from build123d import *

# Parameters (mm, degrees)
SKETCH1_W           = 25.4
SKETCH1_H           = 31.75
BOSS_EXTRUDE1_DEPTH = 25.4
SKETCH2_W           = 3.048
SKETCH2_H           = 19.304
CUT_EXTRUDE1_DEPTH  = 33.534068682
FILLET1_R           = 2.54
CHAMFER1_SIZE       = 1.27


with BuildPart() as part:
    # Sketch1 → Boss-Extrude1 (new body)
    with BuildSketch(Plane(origin=(0, 0, 0), x_dir=(1, 0, 0), z_dir=(0, 1, 0))):
        Rectangle(SKETCH1_W, SKETCH1_H)
    extrude(amount=BOSS_EXTRUDE1_DEPTH)

    # Sketch2 → Cut-Extrude1 (cut, through all)
    with BuildSketch(Plane(origin=(0, 25.4, 0), x_dir=(1, 0, 0), z_dir=(0, 1, 0))):
        with Locations((-4.826, 0)):
            Rectangle(SKETCH2_W, SKETCH2_H)
    extrude(amount=-CUT_EXTRUDE1_DEPTH, mode=Mode.SUBTRACT)

    # Fillet1
    fillet1_edges = [part.edges().sort_by_distance(p)[0] for p in [
        (12.7, 12.7, 15.875),
        (-12.7, 12.7, 15.875),
        (-12.7, 12.7, -15.875),
        (12.7, 12.7, -15.875),
    ]]
    fillet(fillet1_edges, radius=FILLET1_R)

    # Chamfer1
    chamfer1_edges = [part.edges().sort_by_distance(p)[0] for p in [
        (-3.302, 0, 0),
        (-4.826, 0, 9.652),
        (-6.35, 0, 0),
        (-4.826, 0, -9.652),
        (-3.302, 25.4, 0),
        (-4.826, 25.4, -9.652),
        (-6.35, 25.4, 0),
        (-4.826, 25.4, 9.652),
    ]]
    chamfer(chamfer1_edges, length=CHAMFER1_SIZE)


solid = part.part
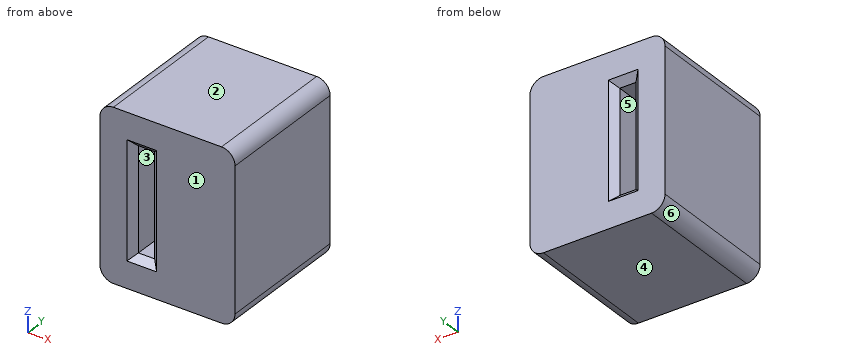
Check sheet for the modelled part. Datum: model origin and axes. Units: mm. Face numbers are marked on the shaded views. A direction names the side the tool comes from. Coordinates: 2 decimals unless noted, no trailing zeros. Loops run counter-clockwise (first coordinate to the right, second up) from the corner with the lowest first, then second, coordinate; pieces in that order, holes last. Notation, with made-up numbers: (-10, 67.5) -> (13, 67.5) arc R23 cw to (13, 94.5) -> close; hole circle Ø8 at (86, -27.5). An arc over 180 degrees is marked (long way). Answer in a Markdown table with one row per item.
1. Material ranges on line 1 along X through (y, z) = (20.5, 6.5); line 2 along Z through (x, y) = (-3.5, 12) (3 decimals); line 3 along X through (y, z) = (11.25, -13.5), recorded low to high. Write a range as [from, to].
Check values:
| item | result |
|---|---|
| line 1 | x = [-12.7, -6.35], [-3.3, 12.7] |
| line 2 | z = [-15.875, -9.652], [9.652, 15.875] |
| line 3 | x = [-12.69, 12.69] |
2. Sectioned sample at B-B, the plane z = -9. Record the boundary of the cut face in (x, y).
Check values:
| item | result |
|---|---|
| outline | (-12.7, 0) -> (-7.62, 0) -> (-6.35, 1.27) -> (-6.35, 24.13) -> (-7.62, 25.4) -> (-12.7, 25.4) -> close; (-3.3, 1.27) -> (-2.03, 0) -> (12.7, 0) -> (12.7, 25.4) -> (-2.03, 25.4) -> (-3.3, 24.13) -> close |
3. Sectioned sample at C-C, the plane x = -6.75. Record the boundary of the cut face in (y, z) (3 decimals).
Check values:
| item | result |
|---|---|
| outline | (0, -15.875) -> (25.4, -15.875) -> (25.4, -10.922) -> (24.53, -10.052) -> (24.53, 10.052) -> (25.4, 10.922) -> (25.4, 15.875) -> (0, 15.875) -> (0, 10.922) -> (0.87, 10.052) -> (0.87, -10.052) -> (0, -10.922) -> close |
4. Release check for a two-part mould opening along Z. For the marked faces 1, 2, 3 and 4 record: released by +Z, released by -Z, zero draft, split by the parting line, or undercut.
Check values:
| item | result |
|---|---|
| face 1 | zero draft |
| face 2 | released by +Z |
| face 3 | undercut |
| face 4 | released by -Z |
5. Sectioned sample at A-A, the plane y = 9.75. Record the boundary of the cut face in (x, z) (3 decimals).
Check values:
| item | result |
|---|---|
| outline | (-12.7, -13.335) arc R2.54 ccw to (-10.16, -15.875) -> (10.16, -15.875) arc R2.54 ccw to (12.7, -13.335) -> (12.7, 13.335) arc R2.54 ccw to (10.16, 15.875) -> (-10.16, 15.875) arc R2.54 ccw to (-12.7, 13.335) -> close; hole (-6.35, -9.652) -> (-3.302, -9.652) -> (-3.302, 9.652) -> (-6.35, 9.652) -> close |
6. Access from +Z, -Z, +X, -X, +Y, -Y to the whole of each face (thin tool, end or side, straight path). Record for the marked faces 5 and 6.
Check values:
| item | result |
|---|---|
| face 5 | +Y, -Y |
| face 6 | -Z, -X, +Y, -Y |
